```python
from build123d import *
from build123d.topology import SkipClean

# Parameters (mm, degrees)
SKETCH1_W           = 32.1
SKETCH1_H           = 12.2
BOSS_EXTRUDE1_DEPTH = 4.3
FILLET1_R           = 0.85
CUT_EXTRUDE1_DEPTH  = 10
SKETCH3_R           = 1
CUT_EXTRUDE2_DEPTH  = 5
BOSS_EXTRUDE2_DEPTH = 4.3
SKETCH6_R           = 4.6
BOSS_EXTRUDE3_DEPTH = 2.4
CUT_EXTRUDE4_DEPTH  = 2.4
SKETCH7_R           = 5.5
BOSS_EXTRUDE4_DEPTH = 2.729404
CUT_EXTRUDE3_DEPTH  = 2.729404426
BOSS_EXTRUDE5_DEPTH = 12.194097
BOSS_EXTRUDE6_DEPTH = 2.82843


with BuildPart() as part:
    # Sketch1 → Boss-Extrude1 (new body)
    with BuildSketch(Plane.XY):
        Rectangle(SKETCH1_W, SKETCH1_H)
    extrude(amount=BOSS_EXTRUDE1_DEPTH)

    # Fillet1
    fillet1_edges = [part.edges().sort_by_distance(p)[0] for p in [
        (16.05, -6.1, 2.15),
        (-16.05, -6.1, 2.15),
        (-16.05, 6.1, 2.15),
        (16.05, 6.1, 2.15),
    ]]
    fillet(fillet1_edges, radius=FILLET1_R)

    # Sketch2 → Cut-Extrude1 (cut)
    with BuildSketch(Plane(origin=(0, 0, 0), x_dir=(-1, 0, 0), z_dir=(0, 0, -1))):
        with BuildLine():
            ThreePointArc((-10.4, 6), (-10.930330086, 5.780330086), (-11.15, 5.25))
            Line((-11.15, 5.25), (-11.15, -5.25))
            ThreePointArc((-11.15, -5.25), (-10.930330086, -5.780330086), (-10.4, -6))
            Line((-10.4, -6), (-10.4, -6.1))
            Line((-10.4, -6.1), (10.4, -6.1))
            Line((10.4, -6.1), (10.4, -6))
            ThreePointArc((10.4, -6), (10.930330086, -5.780330086), (11.15, -5.25))
            Line((11.15, -5.25), (11.15, 5.25))
            ThreePointArc((11.15, 5.25), (10.930330086, 5.780330086), (10.4, 6))
            Line((10.4, 6), (10.4, 6.1))
            Line((10.4, 6.1), (-10.4, 6.1))
            Line((-10.4, 6.1), (-10.4, 6))
        make_face()
        with BuildLine():
            Line((-11.15, -5.25), (-11.15, 5.25))
            ThreePointArc((-11.15, 5.25), (-10.930330086, 5.780330086), (-10.4, 6))
            Line((-10.4, 6), (-10.4, 6.1))
            Line((-10.4, 6.1), (-10.5, 6.1))
            Line((-10.5, 6.1), (-10.5, 6.094097151))
            ThreePointArc((-10.5, 6.094097151), (-11.035413251, 5.81457949), (-11.25, 5.25))
            Line((-11.25, 5.25), (-11.25, -5.25))
            ThreePointArc((-11.25, -5.25), (-11.035413251, -5.81457949), (-10.5, -6.094097151))
            Line((-10.5, -6.094097151), (-10.5, -6.1))
            Line((-10.5, -6.1), (-10.4, -6.1))
            Line((-10.4, -6.1), (-10.4, -6))
            ThreePointArc((-10.4, -6), (-10.930330086, -5.780330086), (-11.15, -5.25))
        make_face()
        with BuildLine():
            Line((10.5, 6.1), (10.4, 6.1))
            Line((10.4, 6.1), (10.4, 6))
            ThreePointArc((10.4, 6), (10.930330086, 5.780330086), (11.15, 5.25))
            Line((11.15, 5.25), (11.15, -5.25))
            ThreePointArc((11.15, -5.25), (10.930330086, -5.780330086), (10.4, -6))
            Line((10.4, -6), (10.4, -6.1))
            Line((10.4, -6.1), (10.5, -6.1))
            Line((10.5, -6.1), (10.5, -6.094097151))
            ThreePointArc((10.5, -6.094097151), (11.035413251, -5.81457949), (11.25, -5.25))
            Line((11.25, -5.25), (11.25, 5.25))
            ThreePointArc((11.25, 5.25), (11.035413251, 5.81457949), (10.5, 6.094097151))
            Line((10.5, 6.094097151), (10.5, 6.1))
        make_face()
    extrude(amount=-CUT_EXTRUDE1_DEPTH, mode=Mode.SUBTRACT)


with BuildPart() as cut_extrude1_piece_1:
    # of the separate pieces the step leaves, piece 1, a body of its own (cut_extrude1_pieces)
    add(part.part.solids().sort_by_distance((-15.2, -6.1, 0))[0])


with BuildPart() as cut_extrude1_piece_2:
    # of the separate pieces the step leaves, piece 2, a body of its own (cut_extrude1_pieces)
    add(part.part.solids().sort_by_distance((10.5, -6.1, 0))[0])


with BuildPart() as cut_extrude2_tool:
    # Sketch3 → Cut-Extrude2 (new body)
    with BuildSketch(Plane.XY.offset(4.3)):
        with Locations((-13.9, 0)):
            Circle(SKETCH3_R)
        with Locations((13.9, 0)):
            Circle(SKETCH3_R)
    extrude(amount=-CUT_EXTRUDE2_DEPTH)


with BuildPart() as cut_extrude1_piece_1_1:
    add(cut_extrude1_piece_1.part)

    # Cut-Extrude2: cut by cut_extrude2_tool
    add(cut_extrude2_tool.part, mode=Mode.SUBTRACT)



with BuildPart() as cut_extrude1_piece_2_1:
    add(cut_extrude1_piece_2.part)

    # Cut-Extrude2: cut by cut_extrude2_tool
    add(cut_extrude2_tool.part, mode=Mode.SUBTRACT)


with BuildPart() as cut_extrude1_piece_1_2:
    add(cut_extrude1_piece_1_1.part)

    add(cut_extrude1_piece_2_1.part)  # Boss-Extrude2 merges Cut-Extrude1 piece 2
    # Sketch5 → Boss-Extrude2 (add)
    with BuildSketch(Plane(origin=(0, 0, 0), x_dir=(-1, 0, 0), z_dir=(0, 0, -1))):
        with BuildLine():
            Line((10.5, 6.1), (10.5, 6.094097151))
            Line((10.5, 6.094097151), (6.291043346, 6.094097151))
            ThreePointArc((6.291043346, 6.094097151), (9.545547959, 4.372545957), (11.25, 1.109053651))
            Line((11.25, 1.109053651), (11.25, -1.109053651))
            ThreePointArc((11.25, -1.109053651), (9.545547959, -4.372545957), (6.291043346, -6.094097151))
            Line((6.291043346, -6.094097151), (10.5, -6.094097151))
            Line((10.5, -6.094097151), (10.5, -6.1))
            Line((10.5, -6.1), (15.2, -6.1))
            ThreePointArc((15.2, -6.1), (15.801040764, -5.851040764), (16.05, -5.25))
            Line((16.05, -5.25), (16.05, 5.25))
            ThreePointArc((16.05, 5.25), (15.801040764, 5.851040764), (15.2, 6.1))
            Line((15.2, 6.1), (10.5, 6.1))
        make_face()
        with BuildLine():
            ThreePointArc((-0.329963504, 2.9), (1.474405208, 4.992995386), (4.008956654, 6.094097151))
            Line((4.008956654, 6.094097151), (-10.5, 6.094097151))
            Line((-10.5, 6.094097151), (-10.5, 6.1))
            Line((-10.5, 6.1), (-15.2, 6.1))
            ThreePointArc((-15.2, 6.1), (-15.801040764, 5.851040764), (-16.05, 5.25))
            Line((-16.05, 5.25), (-16.05, -5.25))
            ThreePointArc((-16.05, -5.25), (-15.801040764, -5.851040764), (-15.2, -6.1))
            Line((-15.2, -6.1), (-10.5, -6.1))
            Line((-10.5, -6.1), (-10.5, -6.094097151))
            Line((-10.5, -6.094097151), (4.008956654, -6.094097151))
            ThreePointArc((4.008956654, -6.094097151), (1.474405208, -4.992995386), (-0.329963504, -2.9))
            Line((-0.329963504, -2.9), (-0.45, -2.9))
            ThreePointArc((-0.45, -2.9), (-3.35, 0), (-0.45, 2.9))
            Line((-0.45, 2.9), (-0.329963504, 2.9))
        make_face()
    extrude(amount=BOSS_EXTRUDE2_DEPTH)

    # Sketch12 → Boss-Extrude5 (add)
    with BuildSketch(Plane.XZ.offset(6.094097151)):
        Polygon((1.05, -7.128427125), (3.878427125, -4.3), (1.05, -4.3), align=None)
        Polygon((-11.25, -6.421320344), (-13.371320344, -4.3), (-11.25, -4.3), align=None)
    extrude(amount=-BOSS_EXTRUDE5_DEPTH)



with BuildPart() as body_2:
    # Sketch6 → Boss-Extrude3 (new body)
    with BuildSketch(Plane(origin=(0, 0, -4.3), x_dir=(-1, 0, 0), z_dir=(0, 0, -1))):
        with BuildLine():
            Line((-0.329963504, -2.9), (-0.45, -2.9))
            ThreePointArc((-0.45, -2.9), (-3.35, 0), (-0.45, 2.9))
            Line((-0.45, 2.9), (-0.329963504, 2.9))
            ThreePointArc((-0.329963504, 2.9), (2.45609555, 5.584163215), (6.291043346, 6.094097151))
            ThreePointArc((6.291043346, 6.094097151), (9.545547959, 4.372545957), (11.25, 1.109053651))
            Line((11.25, 1.109053651), (11.25, -1.109053651))
            ThreePointArc((11.25, -1.109053651), (9.545547959, -4.372545957), (6.291043346, -6.094097151))
            ThreePointArc((6.291043346, -6.094097151), (2.45609555, -5.584163215), (-0.329963504, -2.9))
        make_face()
        with Locations((5.15, 0)):
            Circle(SKETCH6_R, mode=Mode.SUBTRACT)
    extrude(amount=BOSS_EXTRUDE3_DEPTH)

    # Sketch11 → Cut-Extrude4 (cut)
    with BuildSketch(Plane(origin=(0, 0, -6.7), x_dir=(-1, 0, 0), z_dir=(0, 0, -1))):
        with BuildLine():
            ThreePointArc((-0.329963504, -2.9), (-1.05, 0), (-0.329963504, 2.9))
            Line((-0.329963504, 2.9), (-0.45, 2.9))
            ThreePointArc((-0.45, 2.9), (-3.35, 0), (-0.45, -2.9))
            Line((-0.45, -2.9), (-0.329963504, -2.9))
        make_face()
        with BuildLine():
            ThreePointArc((-0.329963504, 2.9), (-0.172147578, 3.180368714), (0, 3.452173229))
            Line((0, 3.452173229), (-4.085462696, 3.186724013))
            Line((-4.085462696, 3.186724013), (-4.085462696, -3.40285267))
            Line((-4.085462696, -3.40285267), (0, -3.452173229))
            ThreePointArc((0, -3.452173229), (-0.172147578, -3.180368714), (-0.329963504, -2.9))
            Line((-0.329963504, -2.9), (-0.45, -2.9))
            ThreePointArc((-0.45, -2.9), (-3.35, 0), (-0.45, 2.9))
            Line((-0.45, 2.9), (-0.329963504, 2.9))
        make_face()
    extrude(amount=-CUT_EXTRUDE4_DEPTH, mode=Mode.SUBTRACT)

    # Sketch7 → Boss-Extrude4 (add)
    with SkipClean():  # the faces are left unmerged after this step: merging them gives an invalid solid
        with BuildSketch(Plane(origin=(0, 0, -6.7), x_dir=(-1, 0, 0), z_dir=(0, 0, -1))):
            with BuildLine():
                Line((11.25, -1.109053651), (11.25, 1.109053651))
                ThreePointArc((11.25, 1.109053651), (6.097619924, 6.127154028), (-0.329963504, 2.9))
                ThreePointArc((-0.329963504, 2.9), (-1.05, 0), (-0.329963504, -2.9))
                ThreePointArc((-0.329963504, -2.9), (6.097619924, -6.127154028), (11.25, -1.109053651))
            make_face()
            with Locations((5.15, 0)):
                Circle(SKETCH7_R, mode=Mode.SUBTRACT)
        extrude(amount=BOSS_EXTRUDE4_DEPTH)

    # Sketch8 → Cut-Extrude3 (cut)
    with SkipClean():  # the faces are left unmerged after this step: merging them gives an invalid solid
        with BuildSketch(Plane(origin=(0, 0, -9.429404426), x_dir=(-1, 0, 0), z_dir=(0, 0, -1))):
            Polygon((9.467113453, 3.407716454), (10.016564256, 3.841425821), (10.016564256, 6.311111289), (0.283435744, 6.311111289), (0.283435744, 3.841425821), (0.832886547, 3.407716454), align=None)
        extrude(amount=-CUT_EXTRUDE3_DEPTH, mode=Mode.SUBTRACT)


with BuildPart() as cut_extrude1_piece_1_3:
    with SkipClean():  # the faces are left unmerged after this step: merging them gives an invalid solid
        add(cut_extrude1_piece_1_2.part)

        add(body_2.part)  # Boss-Extrude6 merges body 2
        # Sketch13 → Boss-Extrude6 (add)
        with BuildSketch(Plane(origin=(0, 0, -4.3), x_dir=(-1, 0, 0), z_dir=(0, 0, -1))):
            with BuildLine():
                Line((4.938256081, 6.19638318), (-1.05, 6.094097151))
                Line((-1.05, 6.094097151), (-1.05, 0))
                ThreePointArc((-1.05, 0), (0.691703672, 4.308548926), (4.938256081, 6.19638318))
            make_face()
            with BuildLine():
                Line((11.25, 6.1), (5.353224073, 6.196668458))
                ThreePointArc((5.353224073, 6.196668458), (9.200137595, 4.694292861), (11.25, 1.109053651))
                Line((11.25, 1.109053651), (11.25, 6.1))
            make_face()
            with BuildLine():
                Line((11.25, -6.094097151), (11.25, -1.109053651))
                ThreePointArc((11.25, -1.109053651), (9.545547959, -4.372545957), (6.291043346, -6.094097151))
                Line((6.291043346, -6.094097151), (10.5, -6.094097151))
                Line((10.5, -6.094097151), (10.5, -6.1))
                Line((10.5, -6.1), (10.909996116, -6.1))
                Line((10.909996116, -6.1), (11.25, -6.094097151))
            make_face()
            with BuildLine():
                ThreePointArc((4.938256081, -6.19638318), (0.691703672, -4.308548926), (-1.05, 0))
                Line((-1.05, 0), (-1.05, -6.094097151))
                Line((-1.05, -6.094097151), (4.938256081, -6.19638318))
            make_face()
        extrude(amount=BOSS_EXTRUDE6_DEPTH)


solid = cut_extrude1_piece_1_3.part
```
CAD build for the part. Positions are in the model's coordinates, mm. A direction names the side the tool comes from. Coordinates: 2 decimals unless noted, no trailing zeros. Order: outer loops, then holes, each group sorted by start corner. A loop starts at its lowest first (then second) coordinate and runs counter-clockwise, first axis right, second up.
(1) Drill centre lines: L1, parallel to Y at x = -13.9, z = 1.05; L2, parallel to Y at x = -5.15, z = -6.15; L3, parallel to Z at x = 4.5, y = 4.25. Where is each one in solid material? Low to high.
Solution:
L1: y = -6.1 to -1, 1 to 6.1
L2: y = -6.2 to -4.6, 4.6 to 6.2
L3: z = -4.3 to 0
(2) Which spindle directions (+Z, -Z, +X, -X, +Y, -Y) get a long thin tool onto all of the face, cutting with end or side? Do faces 4 (the face through (-10, 5, -7.128)), 5 (the face through (2.444, -0.082, -5.734)), 6 (the face through (-2.318, 5.515, -6.911)), 7 (the face through (-10, 5, 0)), 8 (the face through (0, 5, -7.128)). Say none if no direction does.
Solution:
face 4: -Z, -X, +Y
face 5: -Z, +X, +Y, -Y
face 6: -Z
face 7: +Z
face 8: -Z, +X, +Y
(3) Saw through at C-C, the plane x = 13.9. Write the cut outline in (y, z).
Solution:
outline: (-6.1, -4.3) - (6.1, -4.3) - (6.1, 4.3) - (1, 4.3) - (1, 0) - (-1, 0) - (-1, 4.3) - (-6.1, 4.3) - close
(4) Mould opens along Y. For faces 1 (the face through (-12.7, 0.1, 4.3)), 2 (the face through (-13, -6.1, 0)), 3 (the face through (-11.04, 5.81, 2.12)) say: released by +Y, released by -Y, zero draft, split by the parting line, or undercut.
Solution:
face 1: zero draft
face 2: released by -Y
face 3: undercut
(5) Pin check, flat tips, straight feed: pin 1 Ø4.5 at (x, z) = (1, -1.5) entering from +Y; pin 2 Ø4 at (x, y) = (-4, 4) entering from +Z; pin 3 Ø0.6 at (x, y) = (14, 0.5) entering from +Z; pin 4 Ø6 at (x, y) = (-5, 1.5) entering from +Z. Stop position of each tip, or through.
Solution:
pin 1: stops at y = 6.09
pin 2: stops at z = -4.3
pin 3: stops at z = 0
pin 4: passes through
